CAD build for the part. Positions are in the model's coordinates, mm. A direction names the side the tool comes from. Round coordinates to 2 decimals unless told otherwise and drop trailing zeros. Order: outer loops, then holes, each group sorted by start corner. A loop starts at its lowest first (then second) coordinate and runs counter-clockwise, first axis right, second up. Notation, with made-up numbers: (57.5, 69) -> (105.5, 69) arc R29 ccw to (105.5, 99) -> close; hole circle Ø8 at (-10, 76). An arc over 180 degrees is marked (long way). Return JSON: item names as keys, results as strings. Group by question number.
Q1. Cut at D-D (z = 21.5). Write the cut outline in (x, y).
Q2. Which spindle directions (+Z, -Z, +X, -X, +Y, -Y) get a long thin tool onto all of the face, cutting with end or side? Do faces 1 (the flat face through (0, 0, 30)), 2 (the cylindrical face through (-0.867, -3.905, 21.902)). Say none if no direction does.
Q3. Cut at C-C (z = 9). Write the cut outline in (x, y).
Q4. Probe line 1 along Z through (x, y) = (11.5, 11); line 2 along Z through (x, y) = (23, 8); line 3 along X through (y, z) = (11, 4.5). List the from-to ranges inside material, lowest first.
Q5. Flat gauge pins, fed straight in: pin 1 (10 mm diameter, centred on x = -2.5, y = -10, fed in from +Z); pin 2 (3 mm diameter, centred on x = 11.5, y = 8.5, fed in from -Z); pin 3 (10 mm diameter, centred on y = -17, z = 5.5, fed in from +X); pin 4 (1.5 mm diameter, centred on x = -18.5, y = -14, fed in from +Z). Where does each tip first touch, or does it go through?
from build123d import *

# Parameters (mm, degrees)
F0_R     = 25
F2_DEPTH = 5
F1_R     = 4
F3_DEPTH = 30
F4_R     = 10
F5_R     = 4.99999
F6_SIZE  = 1


# Not quite as in the source:
# - a fillet or chamfer is up to 0.001 mm smaller than in the source, because OpenCascade refuses the exact size


with BuildPart() as f2:
    # F0 (on Top) → F2 (new body)
    with BuildSketch(Plane.XY):
        Circle(F0_R)
    extrude(amount=F2_DEPTH)

    # F1 (on face) → F3 (join)
    with BuildSketch(Plane.XY):
        Circle(F1_R)
    extrude(amount=F3_DEPTH)

    # F4
    f4_edges = [f2.edges().sort_by_distance(p)[0] for p in [
        (-4, 0, 5),
    ]]
    fillet(f4_edges, radius=F4_R)

    # F5 (radius 5 in the source; OpenCascade refuses exactly that, so slightly less here)
    f5_edges = [f2.edges().sort_by_distance(p)[0] for p in [
        (-25, 0, 5),
    ]]
    fillet(f5_edges, radius=F5_R)

    # F6
    f6_edges = [f2.edges().sort_by_distance(p)[0] for p in [
        (-4, 0, 30),
    ]]
    chamfer(f6_edges, length=F6_SIZE)


solid = f2.part
Solution:
{
 "1": {"outline": "circle Ø8 at (0, 0)"},
 "2": {"face 1": "+Z, +X, -X, +Y, -Y", "face 2": "+Z"},
 "3": {"outline": "circle Ø12 at (0, 0)"},
 "4": {"line 1": "z = 0 to 5", "line 2": "z = 0 to 2.46", "line 3": "x = -19.26 to 19.26"},
 "5": {"pin 1": "stops at z = 10.06", "pin 2": "stops at z = 0", "pin 3": "stops at x = 20.6", "pin 4": "stops at z = 4.36"}
}
